Source: CAD feature listing. Evaluate the final solid. Frame: model axes, mm. A direction names the side the tool comes from. Round coordinates to 2 decimals unless told otherwise and drop trailing zeros. Order: outer loops, then holes, each group sorted by start corner. A loop starts at its lowest first (then second) coordinate and runs counter-clockwise, first axis right, second up. Notation, with made-up numbers: M 81.5,10 L 129.5,10 A9 ccw 129.5,20 Z; hole C 18.25,88 d5. An arc over 180 degrees is marked long. Answer as CSV lines item,"result". Start each with the question number.
Item 1: Set-up query: faces 1 (the face through (-18, 0, 0)), 2 (the face through (32.5, 12, 0)). Return all of +Z, -Z, +X, -X, +Y, -Y with unobstructed straight access to the full face (end or side cutting, diameter ignored); none if empty.
Item 2: Section query A-A on x = -17.5. Return the cut outline in (y, z).
Item 3: Section query B-B on z = 0. Return the cut outline in (x, y), plus the area to 4 significant figures.
Item 4: Line query: line 1 (Y direction, x = 11.5, z = -2); line 2 (Z direction, x = -17, y = -6); line 3 (Z direction, x = -11, y = -6). Output: solid intervals per line, ascending. Write a range as [from, to].
Item 5: Section query C-C on x = 25.5. Return the cut outline in (y, z), plus the area to 3 significant figures.
Item 6: Pull-direction query (X, two-part tool) for faces 3 (the face through (-22.38, -4.93, 1.08)), 4 (the face through (-9.07, -4.93, -5.38)), 5 (the face through (-32.5, 12, 0)); classes: +X half, -X half, draft (parallel to the pull), parting line (faces both ways), or undercut.
Item 7: Section query D-D on z = -20. Return the cut outline in (x, y), plus the area to 4 significant figures.
Item 8: First-contact query: P1, Ø2, axis at x = -24, z = -13, coming from the -Y side. Flat tip, straight axial feed; report the tip coordinate or a pass-through.
from build123d import *

# Parameters (mm, degrees)
SKETCH1_W           = 65
SKETCH1_H           = 50
BOSS_EXTRUDE1_DEPTH = 25
SKETCH2_R           = 10
SKETCH2_R_2         = 5
BOSS_EXTRUDE2_DEPTH = 10


with BuildPart() as part:
    # Sketch1 → Boss-Extrude1 (new body)
    with BuildSketch(Plane(origin=(0, 0, 0), x_dir=(1, 0, 0), z_dir=(0, 1, 0))):
        Rectangle(SKETCH1_W, SKETCH1_H)
    extrude(amount=BOSS_EXTRUDE1_DEPTH)

    # Sketch2 → Boss-Extrude2 (add)
    with BuildSketch(Plane.XZ):
        with Locations(Location((-17.5, 0, 0), (0, 0, 270))):
            Circle(SKETCH2_R)
        with Locations(Location((-17.5, 0, 0), (0, 0, 270))):
            Circle(SKETCH2_R_2, mode=Mode.SUBTRACT)
    extrude(amount=BOSS_EXTRUDE2_DEPTH)


solid = part.part
Results:
1,face 1,"-Y"
1,face 2,"+Z, -Z, +X, +Y, -Y"
2,outline,"M -10,-10 L 0,-10 L 0,-25 L 25,-25 L 25,25 L 0,25 L 0,10 L -10,10 L -10,5 L 0,5 L 0,-5 L -10,-5 Z"
3,outline,"M -32.5,0 L -27.5,0 L -27.5,-10 L -22.5,-10 L -22.5,0 L -12.5,0 L -12.5,-10 L -7.5,-10 L -7.5,0 L 32.5,0 L 32.5,25 L -32.5,25 Z"
3,area,"1,725 mm^2"
4,line 1,"[0, 25]"
4,line 2,"[-9.99, -4.97], [4.97, 9.99]"
4,line 3,"[-7.6, 7.6]"
5,outline,"M 0,-25 L 25,-25 L 25,25 L 0,25 Z"
5,area,"1,250 mm^2"
6,face 3,"undercut"
6,face 4,"parting line"
6,face 5,"-X half"
7,outline,"M -32.5,0 L 32.5,0 L 32.5,25 L -32.5,25 Z"
7,area,"1,625 mm^2"
8,P1,"y = 0"
